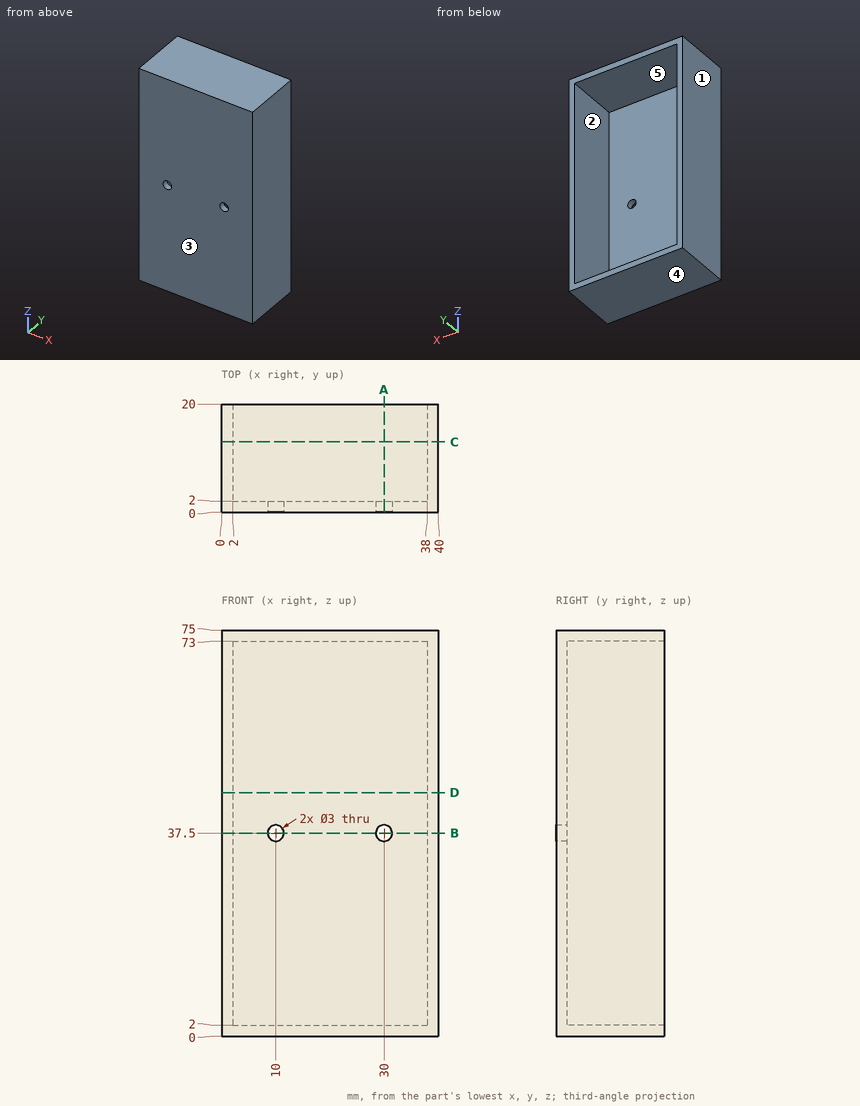
Can you work these out from the drawing? Everything is in mm from the part's minimum corner. A direction names the side the tool comes from. Give positions to 0.01 mm unless a question says otherwise; leave off trailing zeros. Loops run counter-clockwise (first coordinate to the right, second up) from the corner with the lowest first, then second, coordinate; pieces in that order, holes last. Notation, with made-up numbers: (10, 43) - (30, 43) arc R18 ccw to (30, 69) - close; hole circle Ø8 at (16.25, 66). An arc over 180 degrees is marked (long way). Use one line per item in the form item = value.
1. I want a section at C-C (y = 13). Please give me the cut outline in (x, z).
Response values:
outline = (0, 0) - (40, 0) - (40, 75) - (0, 75) - close; hole (2, 2) - (38, 2) - (38, 73) - (2, 73) - close
2. I need wall thicknesses on probe 1 along X at (y, z) = (0.9, 37.5); probe 2 along Z at (x, y) = (29.5, 9.25); probe 3 along Z at (x, y) = (10, 1.55). Which ranges of each line are inside material? Lowest first, please.
Response values:
probe_1 = 0 to 8.5, 11.5 to 28.5, 31.5 to 40
probe_2 = 0 to 2, 73 to 75
probe_3 = 0 to 36, 39 to 75
3. I'm going to push a flat-ended pin straight in: pin 1 Ø3 at (x, z) = (6, 55) entering from +Y. Where does the tip first touch, or does it pass through?
Response values:
pin_1 = 2
4. I want a section at B-B (z = 37.5). Please give me the cut outline in (x, y).
Response values:
outline = (0, 0) - (8.5, 0) - (8.5, 2) - (2, 2) - (2, 20) - (0, 20) - close; (11.5, 0) - (28.5, 0) - (28.5, 2) - (11.5, 2) - close; (31.5, 0) - (40, 0) - (40, 20) - (38, 20) - (38, 2) - (31.5, 2) - close
5. Thinking about a two-plate mould opening in Z: for the marked faces 3, 4 and 5, which applies, released by +Z, released by -Z, zero draft, split by the parting line, or undercut?
Response values:
face_3 = zero draft
face_4 = released by -Z
face_5 = undercut
6. On a 3-axis mill with a long thin cutter (end or side, diameter ignored), from which of +Z, -Z, +X, -X, +Y, -Y can I reach the whole of each face in a straight line? I mean the marked faces 1 and 2. Say none if no direction works.
Response values:
face_1 = +Z, -Z, -X, +Y, -Y
face_2 = +Y
7. I want a section at A-A (x = 30). Please give me the cut outline in (y, z).
Response values:
outline = (0, 0) - (20, 0) - (20, 2) - (2, 2) - (2, 36) - (0, 36) - close; (0, 39) - (2, 39) - (2, 73) - (20, 73) - (20, 75) - (0, 75) - close
8. I want a section at D-D (z = 45). Please give me the cut outline in (x, y).
Response values:
outline = (0, 0) - (40, 0) - (40, 20) - (38, 20) - (38, 2) - (2, 2) - (2, 20) - (0, 20) - close
